Could you check a few things on this drawing? It's one solid part, dimensions in mm from its lowest x, y, z. A direction names the side the tool comes from. Give positions to 0.01 mm unless a question says otherwise; leave off trailing zeros. Order: outer loops, then holes, each group sorted by start corner. A loop starts at its lowest first (then second) coordinate and runs counter-clockwise, first axis right, second up.
Item 1: I want a section at B-B, the plane y = 9.25. Write out the boundary of the cut face in (x, z).
Item 2: I want a section at A-A, the plane z = 3.75. Write out the boundary of the cut face in (x, y).
Item 3: I want a section at D-D, the plane x = 7.5. Write out the boundary of the cut face in (y, z).
Item 4: Which directions (+Z, -Z, +X, -X, +Y, -Y) give clear straight access to the entire face, cutting with the end or side of a thin tool? Please do the marked faces 1, 2, 3 and 4.
Item 5: If I drill on line 1 along X through (y, z) = (1.25, 3); line 2 along X through (y, z) = (0.75, 2.5); line 3 along X through (y, z) = (5.5, 4.75) (1 decimal), over which ranges is the centre line in solid material (lowest first)?
Item 6: I want a section at C-C, the plane x = 3. Write out the boundary of the cut face in (y, z).
Item 7: I'm going to push a flat-ended pin straight in: pin 1 Ø1.5 at (y, z) = (4.5, 6) entering from -X. Where does the tip first touch, or does it pass through?
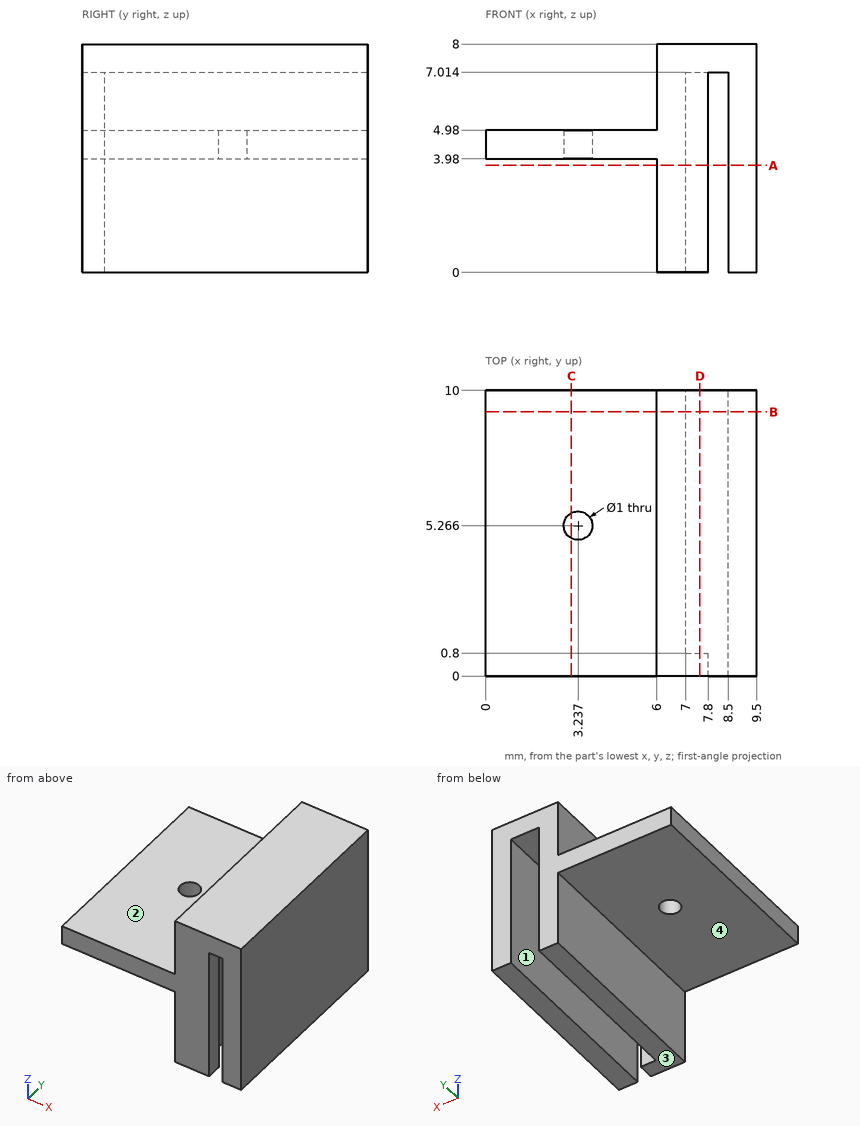
Results list:
1. outline: (0, 3.98) - (6, 3.98) - (6, 0) - (7, 0) - (7, 7.01) - (8.5, 7.01) - (8.5, 0) - (9.5, 0) - (9.5, 8) - (6, 8) - (6, 4.98) - (0, 4.98) - close
2. outline: (6, 0) - (7.8, 0) - (7.8, 0.8) - (7, 0.8) - (7, 10) - (6, 10) - close; (8.5, 0) - (9.5, 0) - (9.5, 10) - (8.5, 10) - close
3. outline: (0, 0) - (0.8, 0) - (0.8, 7.01) - (10, 7.01) - (10, 8) - (0, 8) - close
4. face 1: -Z, +Y, -Y
4. face 2: +Z, -X, +Y, -Y
4. face 3: -Z, +X, -X, +Y, -Y
4. face 4: -Z, -X, +Y, -Y
5. line 1: x = 6 to 7, 8.5 to 9.5
5. line 2: x = 6 to 7.8, 8.5 to 9.5
5. line 3: x = 0 to 2.8, 3.7 to 7, 8.5 to 9.5
6. outline: (0, 3.98) - (4.83, 3.98) - (4.83, 4.98) - (0, 4.98) - close; (5.71, 3.98) - (10, 3.98) - (10, 4.98) - (5.71, 4.98) - close
7. pin 1: stops at x = 6
